```python
from build123d import *

# Parameters (mm, degrees)
BOSS_EXTRUDE1_DEPTH      = 0.125
BOSS_EXTRUDE1_DEPTH_BACK = 0.125
SKETCH1_W                = 5
SKETCH1_H                = 4
SKETCH2_W                = 5
SKETCH2_H                = 4
BOSS_EXTRUDE2_DEPTH      = 0.7
BOSS_EXTRUDE2_TAPER      = 5
SKETCH3_W                = 5
SKETCH3_H                = 4
BOSS_EXTRUDE3_DEPTH      = 0.7
BOSS_EXTRUDE3_TAPER      = 5
CHAMFER1_SIZE            = 0.4
CHAMFER1_SIZE2           = 0.440025147
BOSS_EXTRUDE4_START      = 0.38
BOSS_EXTRUDE4_DEPTH      = 0.51
LPATTERN1_COUNT          = 2
LPATTERN1_PITCH          = 1.27
LPATTERN1_COL_COUNT      = 3
LPATTERN1_COL_PITCH      = 1.27
SKETCH6_R                = 0.356697025
CUT_EXTRUDE1_DEPTH       = 0.02


with BuildPart() as part:
    # Sketch1 → Boss-Extrude1 (new, two sides: drawn at the far end of the back side and taken through both)
    with BuildSketch(Plane(origin=(0, 0.92, 0), x_dir=(1, 0, 0), z_dir=(0, 1, 0)).offset(-BOSS_EXTRUDE1_DEPTH_BACK)):
        Rectangle(SKETCH1_W, SKETCH1_H)
    extrude(amount=BOSS_EXTRUDE1_DEPTH + BOSS_EXTRUDE1_DEPTH_BACK)

    # Sketch2 → Boss-Extrude2 (add)
    with BuildSketch(Plane(origin=(0, 1.045, 0), x_dir=(1, 0, 0), z_dir=(0, 1, 0))):
        Rectangle(SKETCH2_W, SKETCH2_H)
    extrude(amount=BOSS_EXTRUDE2_DEPTH, taper=BOSS_EXTRUDE2_TAPER)

    # Sketch3 → Boss-Extrude3 (add)
    with BuildSketch(Plane.XZ.offset(-0.795)):
        Rectangle(SKETCH3_W, SKETCH3_H)
    extrude(amount=BOSS_EXTRUDE3_DEPTH, taper=BOSS_EXTRUDE3_TAPER)

    # Chamfer1
    chamfer1_edges = [part.edges().sort_by_distance(p)[0] for p in [
        (0, 1.745, 1.938757936),
    ]]
    chamfer1_side = [part.faces().sort_by_distance(p)[0] for p in [
        (0, 1.393553299, 1.969505538),
    ]]
    chamfer(chamfer1_edges, length=CHAMFER1_SIZE, length2=CHAMFER1_SIZE2, reference=chamfer1_side[0])

    # Sketch5 → Boss-Extrude4 (add)
    with BuildSketch(Plane(origin=(0, 0, 0), x_dir=(0, 0, -1), z_dir=(1, 0, 0)).offset(BOSS_EXTRUDE4_START)):
        with BuildLine():
            Line((2.43285762, 0.329963507), (2.38761047, 0.698105953))
            ThreePointArc((2.38761047, 0.698105953), (2.260085254, 0.945612561), (2, 1.045))
            Line((2, 1.045), (2, 0.795))
            ThreePointArc((2, 0.795), (2.091746463, 0.76074775), (2.138599743, 0.674751237))
            Line((2.138599743, 0.674751237), (2.184724748, 0.299466331))
            ThreePointArc((2.184724748, 0.299466331), (2.300209515, 0.080013931), (2.532110769, -0.007837622))
            Line((2.532110769, -0.007837622), (3.099630301, -0.007837622))
            Line((3.099630301, -0.007837622), (3.099630301, 0.242162378))
            Line((3.099630301, 0.242162378), (2.532110769, 0.242162378))
            ThreePointArc((2.532110769, 0.242162378), (2.465853268, 0.267262822), (2.43285762, 0.329963507))
        make_face()
        with BuildLine():
            ThreePointArc((-2.138599743, 0.674751237), (-2.091746463, 0.76074775), (-2, 0.795))
            Line((-2, 0.795), (-2, 1.045))
            ThreePointArc((-2, 1.045), (-2.260085254, 0.945612561), (-2.38761047, 0.698105953))
            Line((-2.38761047, 0.698105953), (-2.43285762, 0.329963507))
            ThreePointArc((-2.43285762, 0.329963507), (-2.465853268, 0.267262822), (-2.532110769, 0.242162378))
            Line((-2.532110769, 0.242162378), (-3.099630301, 0.242162378))
            Line((-3.099630301, 0.242162378), (-3.099630301, -0.007837622))
            Line((-3.099630301, -0.007837622), (-2.532110769, -0.007837622))
            ThreePointArc((-2.532110769, -0.007837622), (-2.300209515, 0.080013931), (-2.184724748, 0.299466331))
            Line((-2.184724748, 0.299466331), (-2.138599743, 0.674751237))
        make_face()
    boss_extrude4 = extrude(amount=BOSS_EXTRUDE4_DEPTH)

    # LPattern1: Boss-Extrude4 ×2
    with Locations(*[(i * LPATTERN1_PITCH, 0, 0) for i in range(1, LPATTERN1_COUNT)]):
        add(boss_extrude4)

    # LPattern1 col: Boss-Extrude4 ×3
    with Locations(*[(-i * LPATTERN1_COL_PITCH, 0, 0) for i in range(1, LPATTERN1_COL_COUNT)]):
        add(boss_extrude4)

    # Sketch6 → Cut-Extrude1 (cut)
    with BuildSketch(Plane(origin=(0, 1.745, 0), x_dir=(1, 0, 0), z_dir=(0, 1, 0))):
        with Locations(Location((-1.829466097, -0.997890598, 0), (0, 0, 270))):
            Circle(SKETCH6_R)
    extrude(amount=-CUT_EXTRUDE1_DEPTH, mode=Mode.SUBTRACT)


solid = part.part
```
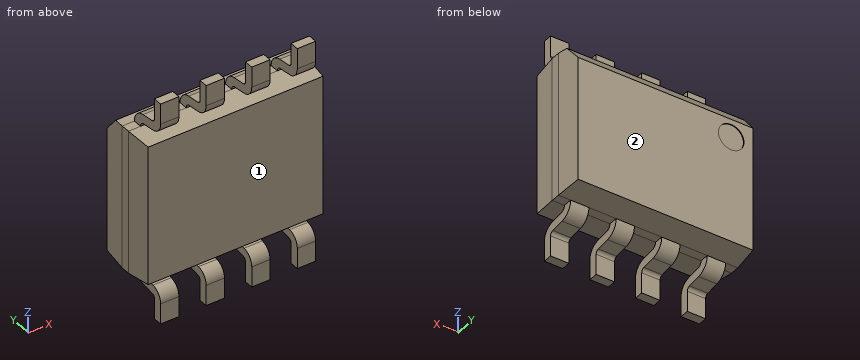
For this review, take the finished solid that the model builds, in its own axes (mm). Face numbers are marked on the shaded views. Coordinates: 2 decimals unless noted, no trailing zeros. Answer in a Markdown table with one row per item. Add a question column.
Q1. For probe 1 along X at (y, z) = (0.2, 2.75); probe 2 along Z at (x, y) = (-1.8, 0.3); probe 3 along X at (y, z) = (1.35, -1.75), list the stretches that pass through material, from the lowest coordinate up.
Q2. Draft analysis for pull direction Z (two halves, no side actions). For the marked faces 1 and 2, state which applies: +Z half, -Z half, draft (parallel to the pull), parting line (faces both ways), or undercut.
Q3. For P1, Ø0.8, axis at y = 0.5, z = 2.5, coming from the -X side; P2, Ø0.6, axis at x = -2, z = 3, coming from the +Y side, all flat-tipped, find the tip position at first contact; note any pin that passes through.
Answer list:
| question | item | result |
|---|---|---|
| 1 | probe 1 | x = -2.16 to -1.65, -0.89 to -0.38, 0.38 to 0.89, 1.65 to 2.16 |
| 1 | probe 2 | z = -2.44 to -2.18, -1.96 to 1.96, 2.18 to 2.44 |
| 1 | probe 3 | x = -2.47 to 2.47 |
| 2 | face 1 | undercut |
| 2 | face 2 | draft |
| 3 | P1 | stops at x = -2.16 |
| 3 | P2 | stops at y = 0.24 |
